Build history of the part. All positions in model axes, mm. A direction names the side the tool comes from. Round coordinates to 2 decimals unless told otherwise and drop trailing zeros. Write each loop counter-clockwise with the first axis right and the second up, starting at its lowest first coordinate (ties: lowest second). Pieces come first, ordered by that corner, then holes.
1) Pull direction Z, two halves, no side cores. Call faces 4 (the cylindrical face through (-65.859, 6.902, 13.793)), 5 (the cylindrical face through (-66.62, -0.78, -41.88)), 6 (the flat face through (-59, 0, 6)), 7 (the flat face through (54, 13, 13)): +Z half, -Z half, draft (parallel to the pull), parting line (faces both ways), or undercut.
2) Saw through at D-D (z = -37). Write the cut outline in (x, y), plus the area to 3 significant figures.
3) Saw through at C-C (y = 1.75). Write the cut outline in (x, z), plus the area to 3 significant figures.
4) Wall check: probe 1 along X at (y, z) = (10.75, -30); probe 2 along X at (y, z) = (2.75, -33); probe 3 along Z at (x, y) = (-17, 7.5). Give the ranges that are in metal, low to high.
5) Saw through at B-B (x = 56). Write the cut outline in (y, z).
6) Saw through at A-A (x = -34.5). Write the cut outline in (y, z), plus the area to 3 significant figures.
7) Flat gauge pins, fed straight in: pin 1 (4 mm diameter, centred on x = -58.63, z = -35.5, fed in from -Y); pin 2 (7.5 mm diameter, centred on x = -58.63, z = 6.5, fed in from +Y); pin 3 (4 mm diameter, centred on x = 63.3, z = -35.5, fed in from +Y). Where does each tip first touch, or does it go through?
8) Which spindle directions (+Z, -Z, +X, -X, +Y, -Y) get a long thin tool onto all of the face, cutting with end or side? Do faces 1 (the cylindrical face through (70.625, 6.902, 13.7)), 2 (the flat face through (-59, 0, -36)), 3 (the flat face through (49.336, 9, 13)). Say none if no direction does.
from build123d import *

# Parameters (mm, degrees)
BOSS_EXTRUDE1_DEPTH = 16
SKETCH2_R           = 3.2
BOSS_EXTRUDE2_DEPTH = 6
SKETCH3_W           = 10
SKETCH3_H           = 7
CUT_EXTRUDE1_DEPTH  = 28
FILLET2_R           = 2
BOSS_EXTRUDE3_DEPTH = 140
FILLET3_R           = 6


with BuildPart() as part:
    # Sketch1 → Boss-Extrude1 (new body)
    with BuildSketch(Plane(origin=(0, 0, 0), x_dir=(1, 0, 0), z_dir=(0, 1, 0))):
        with BuildLine():
            Line((-61.663716814, 44.495575221), (66.336283186, 44.495575221))
            ThreePointArc((66.336283186, 44.495575221), (70.578923873, 42.738215908), (72.336283186, 38.495575221))
            Line((72.336283186, 38.495575221), (72.336283186, -9.504424779))
            ThreePointArc((72.336283186, -9.504424779), (70.578923873, -13.747065466), (66.336283186, -15.504424779))
            Line((66.336283186, -15.504424779), (-61.663716814, -15.504424779))
            ThreePointArc((-61.663716814, -15.504424779), (-65.906357501, -13.747065466), (-67.663716814, -9.504424779))
            Line((-67.663716814, -9.504424779), (-67.663716814, 38.495575221))
            ThreePointArc((-67.663716814, 38.495575221), (-65.906357501, 42.738215908), (-61.663716814, 44.495575221))
        make_face()
        with BuildLine():
            Line((-61.663716814, 40.495575221), (66.336283186, 40.495575221))
            ThreePointArc((66.336283186, 40.495575221), (67.750496748, 39.909788784), (68.336283186, 38.495575221))
            Line((68.336283186, 38.495575221), (68.336283186, -9.504424779))
            ThreePointArc((68.336283186, -9.504424779), (67.750496748, -10.918638341), (66.336283186, -11.504424779))
            Line((66.336283186, -11.504424779), (-61.663716814, -11.504424779))
            ThreePointArc((-61.663716814, -11.504424779), (-63.077930377, -10.918638341), (-63.663716814, -9.504424779))
            Line((-63.663716814, -9.504424779), (-63.663716814, 38.495575221))
            ThreePointArc((-63.663716814, 38.495575221), (-63.077930377, 39.909788784), (-61.663716814, 40.495575221))
        make_face(mode=Mode.SUBTRACT)
    extrude(amount=BOSS_EXTRUDE1_DEPTH)

    # Sketch2 → Boss-Extrude2 (add)
    with BuildSketch(Plane(origin=(0, 0, 0), x_dir=(1, 0, 0), z_dir=(0, 1, 0))):
        with BuildLine():
            Line((-61.663716814, 40.495575221), (66.336283186, 40.495575221))
            ThreePointArc((66.336283186, 40.495575221), (67.750496748, 39.909788784), (68.336283186, 38.495575221))
            Line((68.336283186, 38.495575221), (68.336283186, -9.504424779))
            ThreePointArc((68.336283186, -9.504424779), (67.750496748, -10.918638341), (66.336283186, -11.504424779))
            Line((66.336283186, -11.504424779), (-61.663716814, -11.504424779))
            ThreePointArc((-61.663716814, -11.504424779), (-63.077930377, -10.918638341), (-63.663716814, -9.504424779))
            Line((-63.663716814, -9.504424779), (-63.663716814, 38.495575221))
            ThreePointArc((-63.663716814, 38.495575221), (-63.077930377, 39.909788784), (-61.663716814, 40.495575221))
        make_face()
        with Locations(Location((-58.62788409, 35.495575221, 0), (0, 0, 270))):
            Circle(SKETCH2_R, mode=Mode.SUBTRACT)
        with Locations(Location((63.300450462, 35.495575221, 0), (0, 0, 90))):
            Circle(SKETCH2_R, mode=Mode.SUBTRACT)
        with Locations(Location((-58.62788409, -6.504424779, 0), (0, 0, 90))):
            Circle(SKETCH2_R, mode=Mode.SUBTRACT)
    extrude(amount=BOSS_EXTRUDE2_DEPTH)

    # Sketch3 → Cut-Extrude1 (cut)
    with BuildSketch(Plane.XY):
        with Locations((54.336283186, 9.5)):
            Rectangle(SKETCH3_W, SKETCH3_H)
    extrude(amount=CUT_EXTRUDE1_DEPTH, mode=Mode.SUBTRACT)

    # Fillet2
    fillet2_edges = [part.edges().sort_by_distance(p)[0] for p in [
        (-65.906357501, 16, -42.738215908),
        (-67.663716814, 16, -14.495575221),
        (-65.906357501, 16, 13.747065466),
        (2.336283186, 16, 15.504424779),
        (70.578923873, 16, 13.747065466),
        (72.336283186, 16, -14.495575221),
        (70.578923873, 16, -42.738215908),
        (2.336283186, 16, -44.495575221),
    ]]
    fillet(fillet2_edges, radius=FILLET2_R)

    # Sketch4 → Boss-Extrude3 (add)
    with BuildSketch(Plane(origin=(72.336283186, 0, 0), x_dir=(0, 0, -1), z_dir=(1, 0, 0))):
        Polygon((-15.504424779, 0), (-15.504424779, -11.5), (44.495575221, -1), (44.495575221, 0), align=None)
    extrude(amount=-BOSS_EXTRUDE3_DEPTH)

    # Fillet3
    fillet3_edges = [part.edges().sort_by_distance(p)[0] for p in [
        (-67.663716814, -5.75, 15.504424779),
        (72.336283186, -5.75, 15.504424779),
        (-67.663716814, -0.5, -44.495575221),
        (72.336283186, -0.5, -44.495575221),
    ]]
    fillet(fillet3_edges, radius=FILLET3_R)


solid = part.part
Evaluation:
1. face 4: +Z half
1. face 5: -Z half
1. face 6: undercut
1. face 7: draft
2. outline: (-67.66, -2.31) - (72.34, -2.31) - (72.34, 14) arc R2 ccw to (70.34, 16) - (68.34, 16) - (68.34, 6) - (66.12, 6) - (66.12, 0) - (60.48, 0) - (60.48, 6) - (-55.8, 6) - (-55.8, 0) - (-61.45, 0) - (-61.45, 6) - (-63.66, 6) - (-63.66, 16) - (-65.66, 16) arc R2 ccw to (-67.66, 14) - close
2. area: 1,170 mm2
3. outline: (-67.66, -38.5) arc R6 ccw to (-61.66, -44.5) - (66.34, -44.5) arc R6 ccw to (72.34, -38.5) - (72.34, 9.5) arc R6 ccw to (66.34, 15.5) - (-61.66, 15.5) arc R6 ccw to (-67.66, 9.5) - close; hole circle Ø6.4 at (-58.63, -35.5); hole circle Ø6.4 at (-58.63, 6.5); hole circle Ø6.4 at (63.3, -35.5)
3. area: 8,270 mm2
4. probe 1: x = -67.66 to -63.66, 68.34 to 72.34
4. probe 2: x = -67.66 to -60.63, -56.62 to 61.3, 65.3 to 72.34
4. probe 3: z = -44.5 to -40.5, 11.5 to 15.5
5. outline: (-11.5, 15.5) - (-1, -44.5) - (14, -44.5) arc R2 ccw to (16, -42.5) - (16, -40.5) - (6, -40.5) - (6, 15.5) - close; (13, 11.5) - (16, 11.5) - (16, 13.5) arc R2 ccw to (14, 15.5) - (13, 15.5) - close
6. outline: (-11.5, 15.5) - (-1, -44.5) - (14, -44.5) arc R2 ccw to (16, -42.5) - (16, -40.5) - (6, -40.5) - (6, 11.5) - (16, 11.5) - (16, 13.5) arc R2 ccw to (14, 15.5) - close
6. area: 813 mm2
7. pin 1: stops at y = -2.92
7. pin 2: stops at y = 6
7. pin 3: stops at y = 0
8. face 1: +Z, +X, +Y, -Y
8. face 2: +Y
8. face 3: +Z
